```python
from build123d import *

# Parameters (mm, degrees)
SKETCH1_R           = 8.25
SKETCH1_W           = 9.5
SKETCH1_H           = 3.296
BOSS_EXTRUDE2_DEPTH = 3


with BuildPart() as part:
    # Sketch1 → Boss-Extrude2 (new body)
    with BuildSketch(Plane.XY):
        with BuildLine():
            Line((1.5, 12), (1.5, 10))
            Line((1.5, 10), (-1.5, 10))
            Line((-1.5, 10), (-1.5, 12))
            ThreePointArc((-1.5, 12), (-2.836268406, 12.053611624), (-4.149, 12.309))
            ThreePointArc((-4.149, 12.309), (-17.444023797, 11.979726259), (-22.91780124, -0.140663152))
            ThreePointArc((-22.91780124, -0.140663152), (-20.757463276, -6.337601174), (-15.405, -10.135))
            Line((-15.405, -10.135), (-1.5, -10.135))
            Line((-1.5, -10.135), (-1.5, -5.904))
            Line((-1.5, -5.904), (1.5, -5.904))
            Line((1.5, -5.904), (1.5, -10.135))
            Line((1.5, -10.135), (15.405, -10.135))
            ThreePointArc((15.405, -10.135), (20.757463276, -6.337601174), (22.91780124, -0.140663152))
            ThreePointArc((22.91780124, -0.140663152), (17.444023797, 11.979726259), (4.149, 12.309))
            ThreePointArc((4.149, 12.309), (2.836268406, 12.053611624), (1.5, 12))
        make_face()
        with Locations((-13, 0)):
            Circle(SKETCH1_R, mode=Mode.SUBTRACT)
        with Locations((13, 0)):
            Circle(SKETCH1_R, mode=Mode.SUBTRACT)
        with Locations((0, 7.7)):
            Rectangle(SKETCH1_W, SKETCH1_H, mode=Mode.SUBTRACT)
    extrude(amount=-BOSS_EXTRUDE2_DEPTH)


solid = part.part
```
For this review, take the finished solid that the model builds, in its own axes (mm). A direction names the side the tool comes from. Give positions to 0.01 mm unless a question says otherwise; leave off trailing zeros. Write each loop counter-clockwise with the first axis right and the second up, starting at its lowest first coordinate (ties: lowest second). Pieces come first, ordered by that corner, then holes.
Item 1: Machinability: for faces 1 (the face through (-4.75, 8, -1)), 2 (the face through (8, -10.135, -1)), 3 (the face through (0, -5.904, -1)), 4 (the face through (2.855, 12.056, -1.479)), which of the approach directions +Z, -Z, +X, -X, +Y, -Y give a long, thin tool a straight path to every point of the face, cutting with its end or side? Answer none if there is none.
Item 2: Take a section at A-A (z = -2.55). Give the boundary of the cut face in (x, y) (3 decimals), and give its area (3 significant figures).
Item 3: Take a section at B-B (x = 3.5). Give the boundary of the cut face in (y, z) (3 decimals).
Item 4: Wall thickness on probe 1 along X at (y, z) = (0.5, -2.05); probe 2 along Y at (x, z) = (-1, -0.85); probe 3 along Y at (x, z) = (2, -0.45) (3 decimals): over which ranges is each line inside the solid? List them lowest first.
Item 5: Take a section at C-C (y = 4.5). Give the boundary of the cut face in (x, z), and give its area (3 significant figures).
Item 6: Take a section at D-D (y = 7). Give the boundary of the cut face in (x, z).
Item 7: Insertion check: P1, Ø0.9, axis at y = 7, z = -1.5, coming from the -X side; P2, Ø1.5, axis at x = -2, z = -2, coming from the +Y side; P3, Ø4, axis at x = 12, y = -5.5, coming from the +Z side; P4, Ø1.6, axis at y = 11, z = -2, coming from the +X side. Each pin has a flat end and moves straight along its axis. Give the tip position at first contact, or say it passes through.
Item 8: The part is to be moulded in two halves that separate along Y. For faces 5 (the face through (-9, -10.135, -1)), 6 (the face through (-1.5, -8, -1)), 7 (the face through (0, 6.052, -1)), say which applies: +Y half, -Y half, draft (parallel to the pull), parting line (faces both ways), or undercut.
Established:
1. face 1: +Z, -Z
1. face 2: +Z, -Z, +X, -X, -Y
1. face 3: +Z, -Z, -Y
1. face 4: +Z, -Z, +Y
2. outline: (-22.918, -0.141) arc R10.785 ccw to (-15.405, -10.135) - (-1.5, -10.135) - (-1.5, -5.904) - (1.5, -5.904) - (1.5, -10.135) - (15.405, -10.135) arc R10.785 ccw to (22.918, -0.141) arc R12.5 ccw to (4.149, 12.309) arc R8.804 cw to (1.5, 12) - (1.5, 10) - (-1.5, 10) - (-1.5, 12) arc R8.804 cw to (-4.149, 12.309) arc R12.5 ccw to start; hole circle Ø16.5 at (-13, 0); hole (-4.75, 6.052) - (4.75, 6.052) - (4.75, 9.348) - (-4.75, 9.348) - close; hole circle Ø16.5 at (13, 0)
2. area: 503 mm2
3. outline: (-10.135, -3) - (6.052, -3) - (6.052, 0) - (-10.135, 0) - close; (9.348, -3) - (12.157, -3) - (12.157, 0) - (9.348, 0) - close
4. probe 1: x = -22.99 to -21.23, -4.77 to 4.77, 21.23 to 22.99
4. probe 2: y = -5.9 to 6.05, 9.35 to 10
4. probe 3: y = -10.135 to 6.052, 9.348 to 11.996
5. outline: (-22.68, -3) - (-19.91, -3) - (-19.91, 0) - (-22.68, 0) - close; (-6.09, -3) - (6.09, -3) - (6.09, 0) - (-6.09, 0) - close; (19.91, -3) - (22.68, -3) - (22.68, 0) - (19.91, 0) - close
5. area: 53.1 mm2
6. outline: (-21.79, -3) - (-17.37, -3) - (-17.37, 0) - (-21.79, 0) - close; (-8.63, -3) - (-4.75, -3) - (-4.75, 0) - (-8.63, 0) - close; (4.75, -3) - (8.63, -3) - (8.63, 0) - (4.75, 0) - close; (17.37, -3) - (21.79, -3) - (21.79, 0) - (17.37, 0) - close
7. P1: stops at x = -22
7. P2: stops at y = 12.04
7. P3: passes through
7. P4: stops at x = 19.57
8. face 5: -Y half
8. face 6: draft
8. face 7: undercut
